The model under review builds one solid part; all positions refer to its coordinate system, in mm. Face numbers are marked on the shaded views. Round coordinates to 2 decimals unless told otherwise and drop trailing zeros. Order: outer loops, then holes, each group sorted by start corner. A loop starts at its lowest first (then second) coordinate and runs counter-clockwise, first axis right, second up.
Autodesk Inventor part; units mm, degrees
ref_plane "ip_st_1_1_XY" through (2, 3.75, 0) normal (1, 0, 0) x (0, 0, -1)
ref_plane "ip_st_1_1_YZ" through (2, 3.75, 0) normal (0, 0, -1) x (0, 1, 0)
ref_plane "ip_st_1_1_ZX" through (2, 3.75, 0) normal (0, 1, 0) x (1, 0, 0)
sketch "Sketch_2" plane through (0, 0, 0) normal (0, 0, 1) x (1, 0, 0)
  line L0 (4, 0) -> (0, 0)
  arc A0 (0, 2.15) -> (0.15, 2) centre (0.15, 2.15) ccw
  line L1 (0.15, 2) -> (3.85, 2)
  arc A1 (3.85, 2) -> (4, 2.15) centre (3.85, 2.15) ccw
  line L2 (4, 2.15) -> (4, 2.8)
  line L3 (4, 2.8) -> (3.75, 2.8)
  line L4 (3.75, 2.8) -> (3.75, 3.075)
  line L5 (3.75, 3.075) -> (2.8043, 3.075)
  arc A2 (1.1957, 3.075) -> (2.8043, 3.075) centre (2, 3.75) ccw
  line L6 (1.1957, 3.075) -> (0.25, 3.075)
  line L7 (0.25, 3.075) -> (0.25, 2.8)
  line L8 (0.25, 2.8) -> (0, 2.8)
  line L9 (0, 2.8) -> (0, 2.15)
revolve "Revolution1" add sketch "Sketch_2" angle 360 about axis through (4, 0, 0) along (1, 0, 0)
ref_plane "ip_st_1_1_XY" through (2, 3.75, 0) normal (1, 0, 0) x (0, 0, -1)
ref_plane "ip_st_1_1_YZ" through (2, 3.75, 0) normal (0, 0, -1) x (0, 1, 0)
ref_plane "ip_st_1_1_ZX" through (2, 3.75, 0) normal (0, 1, 0) x (1, 0, 0)
ref_plane "ip_st_1_2_XY" through (2, 2.6517, 2.6517) normal (1, 0, 0) x (0, 0, -1)
ref_plane "ip_st_1_2_YZ" through (2, 2.6517, 2.6517) normal (0, 0, -1) x (0, 1, 0)
ref_plane "ip_st_1_2_ZX" through (2, 2.6517, 2.6517) normal (0, 1, 0) x (1, 0, 0)
ref_plane "ip_st_1_3_XY" through (2, 0, 3.75) normal (1, 0, 0) x (0, 0, -1)
ref_plane "ip_st_1_3_YZ" through (2, 0, 3.75) normal (0, 0, -1) x (0, 1, 0)
ref_plane "ip_st_1_3_ZX" through (2, 0, 3.75) normal (0, 1, 0) x (1, 0, 0)
ref_plane "ip_st_1_4_XY" through (2, -2.6517, 2.6517) normal (1, 0, 0) x (0, 0, -1)
ref_plane "ip_st_1_4_YZ" through (2, -2.6517, 2.6517) normal (0, 0, -1) x (0, 1, 0)
ref_plane "ip_st_1_4_ZX" through (2, -2.6517, 2.6517) normal (0, 1, 0) x (1, 0, 0)
ref_plane "ip_st_1_5_XY" through (2, -3.75, 0) normal (1, 0, 0) x (0, 0, -1)
ref_plane "ip_st_1_5_YZ" through (2, -3.75, 0) normal (0, 0, -1) x (0, 1, 0)
ref_plane "ip_st_1_5_ZX" through (2, -3.75, 0) normal (0, 1, 0) x (1, 0, 0)
ref_plane "ip_st_1_6_XY" through (2, -2.6517, -2.6517) normal (1, 0, 0) x (0, 0, -1)
ref_plane "ip_st_1_6_YZ" through (2, -2.6517, -2.6517) normal (0, 0, -1) x (0, 1, 0)
ref_plane "ip_st_1_6_ZX" through (2, -2.6517, -2.6517) normal (0, 1, 0) x (1, 0, 0)
ref_plane "ip_st_1_7_XY" through (2, 0, -3.75) normal (1, 0, 0) x (0, 0, -1)
ref_plane "ip_st_1_7_YZ" through (2, 0, -3.75) normal (0, 0, -1) x (0, 1, 0)
ref_plane "ip_st_1_7_ZX" through (2, 0, -3.75) normal (0, 1, 0) x (1, 0, 0)
ref_plane "ip_st_1_8_XY" through (2, 2.6517, -2.6517) normal (1, 0, 0) x (0, 0, -1)
ref_plane "ip_st_1_8_YZ" through (2, 2.6517, -2.6517) normal (0, 0, -1) x (0, 1, 0)
ref_plane "ip_st_1_8_ZX" through (2, 2.6517, -2.6517) normal (0, 1, 0) x (1, 0, 0)
ref_plane "ip_st_1a_XY" through (0, 0, 0) normal (1, 0, 0) x (0, 0, -1)
ref_plane "ip_st_1a_YZ" through (0, 0, 0) normal (0, 0, -1) x (0, 1, 0)
ref_plane "ip_st_1a_ZX" through (0, 0, 0) normal (0, 1, 0) x (1, 0, 0)
ref_plane "ip_st_2a_XY" through (0.25, 0, 0) normal (1, 0, 0) x (0, 0, -1)
ref_plane "ip_st_2a_YZ" through (0.25, 0, 0) normal (0, 0, -1) x (0, 1, 0)
ref_plane "ip_st_2a_ZX" through (0.25, 0, 0) normal (0, 1, 0) x (1, 0, 0)
properties part number "F694ZZ Inner Ring" material "ステンレス鋼 440C"
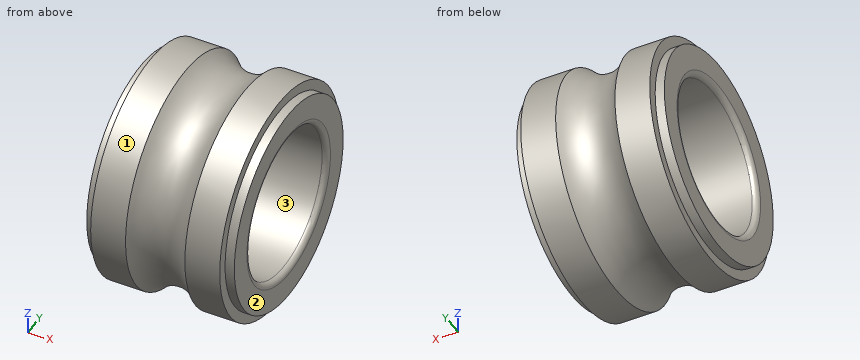
(1) Consider section C-C (x = 3.35). Write out the cut boundary in (y, z) (3 decimals).
Data:
outline: circle Ø6.15 at (0, 0); hole circle Ø4 at (0, 0)
(2) Insertion check: pin 1 (1 mm diameter, centred on y = -1, z = -1, fed in from +X); pin 2 (2 mm diameter, centred on x = 2.5, z = -1.5, fed in from +Y). Each pin has a flat end and moves straight along its axis. Give the tip position at first contact, or say it passes through.
Data:
pin 1: passes through
pin 2: stops at y = 3.03
(3) To check wall thickness, follow probe 1 along Z at (x, y) = (3.05, 0) (3 decimals); probe 2 along Z at (x, y) = (1.7, 0); probe 3 along X at (y, z) = (-2.25, 1.75). State the ranges of each line that lie inside material, in increasing order.
Data:
probe 1: z = -3.075 to -2, 2 to 3.075
probe 2: z = -2.74 to -2, 2 to 2.74
probe 3: x = 0.25 to 1.46, 2.54 to 3.75
(4) Draft analysis for pull direction Z (two halves, no side actions). For the marked faces 1, 2 and 3, state which applies: pulls with the +Z half, pulls with the -Z half, needs draft (parallel to the pull), parting line crosses it, or undercut.
Data:
face 1: parting line crosses it
face 2: needs draft
face 3: undercut
(5) Consider section D-D (x = 2.05). Write out the cut boundary in (y, z).
Data:
outline: circle Ø5.4 at (0, 0); hole circle Ø4 at (0, 0)
(6) Consider section A-A (y = 0). Write out the cut boundary in (x, z) (3 decimals).
Data:
outline: (0, -2.8) - (0.25, -2.8) - (0.25, -3.075) - (1.196, -3.075) arc R1.05 cw to (2.804, -3.075) - (3.75, -3.075) - (3.75, -2.8) - (4, -2.8) - (4, -2.15) arc R0.15 ccw to (3.85, -2) - (0.15, -2) arc R0.15 ccw to (0, -2.15) - close; (0, 2.15) arc R0.15 ccw to (0.15, 2) - (3.85, 2) arc R0.15 ccw to (4, 2.15) - (4, 2.8) - (3.75, 2.8) - (3.75, 3.075) - (2.804, 3.075) arc R1.05 cw to (1.196, 3.075) - (0.25, 3.075) - (0.25, 2.8) - (0, 2.8) - close
